Build history of the part. All positions in model axes, mm. A direction names the side the tool comes from. Give positions to 0.01 mm unless a question says otherwise; leave off trailing zeros. Order: outer loops, then holes, each group sorted by start corner. A loop starts at its lowest first (then second) coordinate and runs counter-clockwise, first axis right, second up. Notation, with made-up numbers: (79, 56.25) - (108, 56.25) arc R23 cw to (108, 73.25) - close; hole circle Ø8 at (65.5, 25.5). An arc over 180 degrees is marked (long way). One line per item, written item: value.
```python
from build123d import *

# Parameters (mm, degrees)
F0_W     = 6.35
F0_H     = 6.35
F1_DEPTH = 177.8
F2_DEPTH = 6.35


with BuildPart() as f1:
    # F0 (on Top) → F1 (new body)
    with BuildSketch(Plane.XY):
        Polygon((9.525, -42.8625), (-9.525, -42.8625), (-3.175, -61.831036), (3.175, -61.831036), align=None)
        with Locations((0, -65.006036)):
            Rectangle(F0_W, F0_H)
    extrude(amount=F1_DEPTH)

    # F0 (on Top) → F2 (join)
    with BuildSketch(Plane.XY):
        with Locations((0, -71.356036)):
            Rectangle(F0_W, F0_H)
    extrude(amount=F2_DEPTH)


solid = f1.part
```
(1) Drill centre lines: line 1 (Y direction, x = 0.5, z = 147); line 2 (X direction, y = -66.5, z = 114.5) (3 decimals); line 3 (X direction, y = -49, z = 154). Where is each one in solid material? Low to high.
Completed:
line 1: -68.18 to -42.86
line 2: -3.175 to 3.175
line 3: -7.47 to 7.47
(2) Slice it at A-A, the plane x = -1. Give the cut face in (y, z).
Completed:
outline: (-74.53, 0) - (-42.86, 0) - (-42.86, 177.8) - (-68.18, 177.8) - (-68.18, 6.35) - (-74.53, 6.35) - close
(3) 3-axis set-ups, long thin cutter, end or side, ignore diameter. For faces 1 (the face through (0, -53, 177.8)), 2 (the face through (-3.175, -64, 88)), 3 (the face through (0, -71, 6.35)), 4 (the face through (3.175, -64, 88)), 5 (the face through (0, -55, 0)): which of +Z, -Z, +X, -X, +Y, -Y reach the whole face in a straight line?
Completed:
face 1: +Z, +X, -X, +Y, -Y
face 2: +Z, -Z, -X, -Y
face 3: +Z, +X, -X, -Y
face 4: +Z, -Z, +X, -Y
face 5: -Z, +X, -X, +Y, -Y
(4) Slice it at D-D, the plane y = -49.5. Give the cut face in (x, z), and give its area (3 significant figures).
Completed:
outline: (-7.3, 0) - (7.3, 0) - (7.3, 177.8) - (-7.3, 177.8) - close
area: 2,600 mm²
(5) Slice it at B-B, the plane z = 33. Give the cut face in (x, y) (1 decimal), and give its area (3 significant figures).
Completed:
outline: (-9.5, -42.9) - (-3.2, -61.8) - (-3.2, -68.2) - (3.2, -68.2) - (3.2, -61.8) - (9.5, -42.9) - close
area: 281 mm²
(6) Slice it at C-C, the plane y = -59. Give the cut face in (x, z), and give its area (3 significant figures).
Completed:
outline: (-4.12, 0) - (4.12, 0) - (4.12, 177.8) - (-4.12, 177.8) - close
area: 1,470 mm²
(7) Pin check, flat tips, straight feed: P1, Ø3, axis at x = 2, z = 154.5, coming from the -Y side; P2, Ø8, axis at y = -63, z = 132, coming from the -X side; P3, Ø4, axis at y = -68.5, z = 58, coming from the +X side (3 decimals). Stop position of each tip, or through.
Completed:
P1: y = -68.18
P2: x = -4.12
P3: x = 3.175
